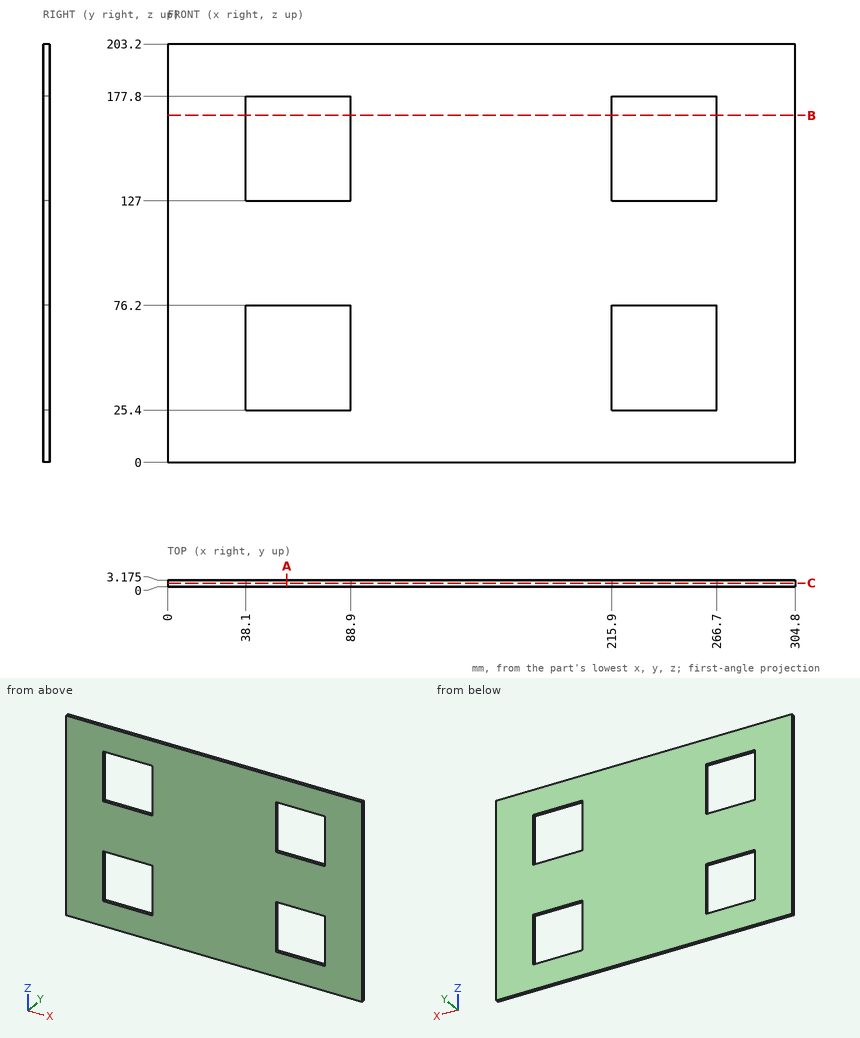
Verification items for this drawing (mm, ordinates from the low corner). Give positions to 0.01 mm unless a question says otherwise; leave off trailing zeros. Write each loop counter-clockwise with the first axis right and the second up, starting at its lowest first coordinate (ties: lowest second). Pieces come first, ordered by that corner, then holes. Notation, with made-up numbers: (23.25, -9) -> (64.25, -9) arc R30 ccw to (64.25, 18) -> close; hole circle Ø4 at (-6, -5.5). An arc over 180 degrees is marked (long way). Use one line per item in the form item = value.
Item 1: Sectioned sample at C-C on y = 1.8. Enter the section's corners in (x, z), plus the area to 3 significant figures.
Results list:
outline = (0, 0) -> (304.8, 0) -> (304.8, 203.2) -> (0, 203.2) -> close; hole (38.1, 25.4) -> (88.9, 25.4) -> (88.9, 76.2) -> (38.1, 76.2) -> close; hole (38.1, 127) -> (88.9, 127) -> (88.9, 177.8) -> (38.1, 177.8) -> close; hole (215.9, 25.4) -> (266.7, 25.4) -> (266.7, 76.2) -> (215.9, 76.2) -> close; hole (215.9, 127) -> (266.7, 127) -> (266.7, 177.8) -> (215.9, 177.8) -> close
area = 51,600 mm2
Item 2: Sectioned sample at A-A on x = 58. Enter the section's corners in (y, z) (3 decimals).
Results list:
outline = (0, 0) -> (3.175, 0) -> (3.175, 25.4) -> (0, 25.4) -> close; (0, 76.2) -> (3.175, 76.2) -> (3.175, 127) -> (0, 127) -> close; (0, 177.8) -> (3.175, 177.8) -> (3.175, 203.2) -> (0, 203.2) -> close
Item 3: Sectioned sample at B-B on z = 168.5. Enter the section's corners in (x, y) (3 decimals).
Results list:
outline = (0, 0) -> (38.1, 0) -> (38.1, 3.175) -> (0, 3.175) -> close; (88.9, 0) -> (215.9, 0) -> (215.9, 3.175) -> (88.9, 3.175) -> close; (266.7, 0) -> (304.8, 0) -> (304.8, 3.175) -> (266.7, 3.175) -> close
Item 4: Scan lines: line 1 (X direction, y = 1.15, z = 147); line 2 (Z direction, x = 54, y = 3). Record each from-to range of solid material in increasing order.
Results list:
line_1 = 0 to 38.1, 88.9 to 215.9, 266.7 to 304.8
line_2 = 0 to 25.4, 76.2 to 127, 177.8 to 203.2
